Autodesk Inventor part; units mm, degrees
ref_plane "YZ Plane" through (0, 0, 0) normal (1, 0, 0) x (0, 1, 0)
ref_plane "XZ Plane" through (0, 0, 0) normal (0, 1, 0) x (-1, 0, 0)
ref_plane "XY Plane" through (0, 0, 0) normal (0, 0, 1) x (1, 0, 0)
sketch "Sketch1" plane through (0, 0, 0) normal (0, 0, 1) x (1, 0, 0)
  line L0 (49.9396, 9.6174) -> (57.9396, 9.6174)
  line L1 (57.9396, -8.4526) -> (49.9396, -8.4526)
  line L2 (49.9396, -8.4526) -> (49.9396, 9.6174)
  line L3 (57.9396, -8.4526) -> (57.9396, 9.6174)
  line L4 (-49.449, 9.6174) -> (-49.449, -8.4526)
  line L5 (-49.449, -8.4526) -> (-57.449, -8.4526)
  line L6 (-57.449, 9.6174) -> (-57.449, -8.4526)
  line L7 (-45.5464, 0.7392) -> (-34.5464, 0.7392)
  line L8 (-33.5464, 1.7392) -> (-33.5464, 6.2392)
  line L9 (-34.5464, 7.2392) -> (-45.5464, 7.2392)
  line L10 (-46.5464, 6.2392) -> (-46.5464, 1.7392)
  line L11 (-30.5291, -2.0275) -> (3.4709, -2.0275)
  line L12 (4.4709, -1.0275) -> (4.4709, 3.9725)
  line L13 (-31.5291, 3.9725) -> (-31.5291, -1.0275)
  circle A0 centre (-88.9996, -15.383) radius 1.5
  circle A1 centre (-64.9996, -15.383) radius 1.5
  circle A2 centre (-64.9996, 8.617) radius 1.5
  circle A3 centre (-88.9996, 8.617) radius 1.5
  arc A4 (-82.1595, 3.0543) -> (-82.1595, -9.8202) centre (-76.9996, -3.383) ccw
  arc A5 (-79.9944, -11.0702) -> (-68.8448, -4.633) centre (-76.9996, -3.383) ccw
  arc A6 (-68.8448, -2.133) -> (-79.9944, 4.3043) centre (-76.9996, -3.383) ccw
  arc A7 (-82.0034, -16.8856) -> (-62.804, -5.8009) centre (-76.9996, -3.383) ccw
  arc A8 (-63.7898, -2.133) -> (-62.804, -0.9651) centre (-63.7898, -1.133) ccw
  arc A9 (-62.804, -0.9651) -> (-82.0034, 10.1197) centre (-76.9996, -3.383) ccw
  arc A10 (-82.0034, 10.1197) -> (-82.5219, 8.682) centre (-81.6559, 9.182) ccw
  line L14 (-82.5219, 8.682) -> (-79.9944, 4.3043)
  line L15 (-82.1595, 3.0543) -> (-84.687, 7.432)
  arc A11 (-84.687, 7.432) -> (-86.1913, 7.7018) centre (-85.553, 6.932) ccw
  arc A12 (-86.1913, 7.7018) -> (-86.1913, -14.4677) centre (-76.9996, -3.383) ccw
  arc A13 (-86.1913, -14.4677) -> (-84.687, -14.1979) centre (-85.553, -13.6979) ccw
  line L16 (-84.687, -14.1979) -> (-82.1595, -9.8202)
  arc A14 (-82.5219, -15.4479) -> (-82.0034, -16.8856) centre (-81.6559, -15.9479) ccw
  line L17 (-79.9944, -11.0702) -> (-82.5219, -15.4479)
  line L18 (-63.7898, -4.633) -> (-68.8448, -4.633)
  arc A15 (-62.804, -5.8009) -> (-63.7898, -4.633) centre (-63.7898, -5.633) ccw
  line L19 (-68.8448, -2.133) -> (-63.7898, -2.133)
  circle A16 centre (64.9975, -15.3839) radius 1.5
  circle A17 centre (88.9975, -15.3839) radius 1.5
  circle A18 centre (88.9975, 8.6161) radius 1.5
  circle A19 centre (64.9975, 8.6161) radius 1.5
  line L20 (71.4751, 8.6811) -> (74.0026, 4.3033)
  arc A20 (71.9936, 10.1188) -> (71.4751, 8.6811) centre (72.3411, 9.1811) ccw
  arc A21 (91.193, -0.966) -> (71.9936, 10.1188) centre (76.9975, -3.3839) ccw
  arc A22 (85.1522, -2.1339) -> (74.0026, 4.3033) centre (76.9975, -3.3839) ccw
  line L21 (85.1522, -2.1339) -> (90.2072, -2.1339)
  arc A23 (90.2072, -2.1339) -> (91.193, -0.966) centre (90.2072, -1.1339) ccw
  arc A24 (91.193, -5.8018) -> (90.2072, -4.6339) centre (90.2072, -5.6339) ccw
  arc A25 (71.9936, -16.8866) -> (91.193, -5.8018) centre (76.9975, -3.3839) ccw
  arc A26 (74.0026, -11.0711) -> (85.1522, -4.6339) centre (76.9975, -3.3839) ccw
  line L22 (74.0026, -11.0711) -> (71.4751, -15.4489)
  line L23 (69.31, -14.1989) -> (71.8375, -9.8211)
  arc A27 (67.8057, -14.4686) -> (69.31, -14.1989) centre (68.444, -13.6989) ccw
  arc A28 (67.8057, 7.7009) -> (67.8057, -14.4686) centre (76.9975, -3.3839) ccw
  arc A29 (71.8375, 3.0533) -> (71.8375, -9.8211) centre (76.9975, -3.3839) ccw
  line L24 (71.8375, 3.0533) -> (69.31, 7.4311)
  arc A30 (69.31, 7.4311) -> (67.8057, 7.7009) centre (68.444, 6.9311) ccw
  arc A31 (71.4751, -15.4489) -> (71.9936, -16.8866) centre (72.3411, -15.9489) ccw
  line L25 (90.2072, -4.6339) -> (85.1522, -4.6339)
  line L26 (-49.449, 9.6174) -> (-57.449, 9.6174)
  line L27 (3.4709, 4.9725) -> (-30.5291, 4.9725)
  arc A32 (-34.5464, 0.7392) -> (-33.5464, 1.7392) centre (-34.5464, 1.7392) ccw
  arc A33 (-33.5464, 6.2392) -> (-34.5464, 7.2392) centre (-34.5464, 6.2392) ccw
  arc A34 (-45.5464, 7.2392) -> (-46.5464, 6.2392) centre (-45.5464, 6.2392) ccw
  arc A35 (-46.5464, 1.7392) -> (-45.5464, 0.7392) centre (-45.5464, 1.7392) ccw
  arc A36 (-31.5291, -1.0275) -> (-30.5291, -2.0275) centre (-30.5291, -1.0275) ccw
  arc A37 (-30.5291, 4.9725) -> (-31.5291, 3.9725) centre (-30.5291, 3.9725) ccw
  arc A38 (4.4709, 3.9725) -> (3.4709, 4.9725) centre (3.4709, 3.9725) ccw
  arc A39 (3.4709, -2.0275) -> (4.4709, -1.0275) centre (3.4709, -1.0275) ccw
  line L28 (-57.412, 19.6174) -> (-87.412, 19.6174)
  line L29 (-87.412, 19.6174) -> (-87.412, 24.6174)
  line L30 (-57.412, 24.6174) -> (-87.412, 24.6174)
  line L31 (-57.412, 19.6174) -> (-57.412, 24.6174)
  line L32 (27.588, 19.6174) -> (-27.412, 19.6174)
  line L33 (-27.412, 19.6174) -> (-27.412, 24.6174)
  line L34 (27.588, 24.6174) -> (-27.412, 24.6174)
  line L35 (27.588, 19.6174) -> (27.588, 24.6174)
  line L36 (87.588, 19.6174) -> (57.588, 19.6174)
  line L37 (57.588, 19.6174) -> (57.588, 24.6174)
  line L38 (87.588, 24.6174) -> (57.588, 24.6174)
  line L39 (87.588, 19.6174) -> (87.588, 24.6174)
  line L40 (94.088, -10.3826) -> (94.088, -25.3826)
  line L41 (99.088, -10.3826) -> (94.088, -10.3826)
  line L42 (99.088, 9.6181) -> (99.088, -10.3826)
  line L43 (99.088, 9.6181) -> (94.088, 9.6181)
  line L44 (94.088, 24.6181) -> (94.088, 9.6181)
  line L45 (99.088, 24.6181) -> (94.088, 24.6181)
  line L46 (99.088, 32.6174) -> (99.088, 24.6181)
  line L47 (-98.912, 32.6174) -> (-98.912, 24.6181)
  line L48 (-93.912, 24.6181) -> (-98.912, 24.6181)
  line L49 (-93.912, 24.6181) -> (-93.912, 9.6181)
  line L50 (-93.912, 9.6181) -> (-98.912, 9.6181)
  line L51 (-98.912, 9.6181) -> (-98.912, -10.3826)
  line L52 (-93.912, -10.3826) -> (-98.912, -10.3826)
  line L53 (-93.912, -10.3826) -> (-93.912, -25.3826)
  line L54 (-98.912, 32.6174) -> (99.088, 32.6174)
  line L55 (-93.912, -25.3826) -> (94.088, -25.3826)
  arc A40 (15.5314, -3.6707) -> (16.5314, -2.6707) centre (15.5314, -2.6707) ccw
  arc A41 (16.5314, 5.8293) -> (15.5314, 6.8293) centre (15.5314, 5.8293) ccw
  line L56 (5.7314, -2.6707) -> (5.7314, 5.8293)
  arc A42 (5.7314, -2.6707) -> (6.7314, -3.6707) centre (6.7314, -2.6707) ccw
  arc A43 (6.7314, 6.8293) -> (5.7314, 5.8293) centre (6.7314, 5.8293) ccw
  line L57 (6.7314, 6.8293) -> (15.5314, 6.8293)
  line L58 (6.7314, -3.6707) -> (15.5314, -3.6707)
  line L59 (23.4252, 0.4179) -> (23.4252, -9.0821)
  line L60 (37.4252, 1.4179) -> (24.4252, 1.4179)
  line L61 (24.4252, -10.0821) -> (37.4252, -10.0821)
  line L62 (38.4252, -9.0821) -> (38.4252, 0.4179)
  line L63 (16.5314, -2.6707) -> (16.5314, 5.8293)
  arc A44 (24.4252, 1.4179) -> (23.4252, 0.4179) centre (24.4252, 0.4179) ccw
  arc A45 (23.4252, -9.0821) -> (24.4252, -10.0821) centre (24.4252, -9.0821) ccw
  arc A46 (37.4252, -10.0821) -> (38.4252, -9.0821) centre (37.4252, -9.0821) ccw
  arc A47 (38.4252, 0.4179) -> (37.4252, 1.4179) centre (37.4252, 0.4179) ccw
  point P0 (-50.5662, -19.8134)
  point P1 (94.0004, -33.3808)
  point P2 (-46.5464, 0.7392)
  point P3 (-33.5464, 7.2392)
  point P4 (-33.5464, 0.7392)
  point P5 (-46.5464, 7.2392)
  point P6 (-31.5291, -2.0275)
  point P7 (4.4709, 4.9725)
  point P8 (4.4709, -2.0275)
  point P9 (-31.5291, 4.9725)
  point P10 (3.4709, -1.0275)
  point P11 (23.4252, 1.4179)
  point P12 (5.7314, -3.6707)
  point P13 (16.5314, 6.8293)
  point P14 (16.5314, -3.6707)
  point P15 (23.4252, -10.0821)
  point P16 (38.4252, -10.0821)
  point P17 (38.4252, 1.4179)
  dimension "d20" = 8
  dimension "d47" = 8
  dimension "d53" = 6.5
  dimension "d54" = 13
  dimension "d56" = 36
  dimension "d59" = 1
  dimension "d60" = 7
  dimension "d73" = 10.5
  dimension "d74" = 10.8
  dimension "d75" = 11.5
  dimension "d76" = 15
extrude "Extrusion2" add sketch "Sketch1" along normal blind 5
sketch "Sketch2" plane through (0, 0, 0) normal (0, 0, -1) x (-1, 0, 0)
  line L0 (92.3846, -19.3253) -> (61.6146, -19.3253)
  line L1 (61.6146, -19.3253) -> (61.6146, 12.5593)
  line L2 (61.6146, 12.5593) -> (92.3846, 12.5593)
  line L3 (92.3846, 12.5593) -> (92.3846, -19.3253)
  arc A0 (82.1595, -9.8202) -> (82.1595, 3.0543) centre (76.9996, -3.383) ccw
  line L4 (92.3846, -19.3253) -> (61.6146, 12.5593) construction
  line L5 (61.6146, -19.3253) -> (92.3846, 12.5593) construction
  line L6 (-61.3514, -21.1002) -> (-92.6435, -21.1002)
  line L7 (-92.6435, -21.1002) -> (-92.6435, 14.3324)
  line L8 (-92.6435, 14.3324) -> (-61.3514, 14.3324)
  line L9 (-61.3514, 14.3324) -> (-61.3514, -21.1002)
  arc A1 (-67.8057, -14.4686) -> (-67.8057, 7.7009) centre (-76.9975, -3.3839) ccw
  line L10 (-61.3514, -21.1002) -> (-92.6435, 14.3324) construction
  line L11 (-92.6435, -21.1002) -> (-61.3514, 14.3324) construction
  point P0 (0, 0)
extrude "Extrusion3" add sketch "Sketch2" against normal blind 5
sketch "Sketch3" plane through (0, 0, 0) normal (0, 0, -1) x (-1, 0, 0)
  line L0 (44.362, -11.7916) -> (-44.638, -11.7916)
  line L1 (-48.638, -7.7916) -> (-48.638, 6.2084)
  line L2 (-44.638, 10.2084) -> (44.362, 10.2084)
  line L3 (48.362, 6.2084) -> (48.362, -7.7916)
  line L4 (48.362, -11.7916) -> (-48.638, 10.2084) construction
  line L5 (-48.638, -11.7916) -> (48.362, 10.2084) construction
  arc A0 (44.362, -11.7916) -> (48.362, -7.7916) centre (44.362, -7.7916) ccw
  arc A1 (-48.638, -7.7916) -> (-44.638, -11.7916) centre (-44.638, -7.7916) ccw
  arc A2 (-44.638, 10.2084) -> (-48.638, 6.2084) centre (-44.638, 6.2084) ccw
  arc A3 (48.362, 6.2084) -> (44.362, 10.2084) centre (44.362, 6.2084) ccw
  line L6 (-99.088, -10.3826) -> (-99.088, 9.6181)
  line L7 (-99.088, 32.6174) -> (98.912, 32.6174)
  line L8 (98.912, 9.6181) -> (98.912, -10.3826)
  point P0 (0, 0)
  point P1 (-0.138, -0.7916)
  point P2 (-48.638, -0.7916)
  dimension "d79" = 97
  dimension "d80" = 22
  dimension "d81" = 4
  dimension "d83" = 22.409
  dimension "d84" = 50.55
extrude "Extrusion4" cut sketch "Sketch3" against normal blind 5
properties part number "case top back" material "Lead"
Here's how the part is built. I have some questions about the finished solid (model axes, mm). A direction names the side the tool comes from. Give positions to 0.01 mm unless a question says otherwise; leave off trailing zeros. Loops run counter-clockwise (first coordinate to the right, second up) from the corner with the lowest first, then second, coordinate; pieces in that order, holes last. Notation, with made-up numbers: M 36,21.5 L 82,21.5 A12 cw 82,42.5 Z; hole C 24,49 d6. An arc over 180 degrees is marked long. Use one line per item in the form item = value. Start each with the question number.
Q1. If we section it at C-C (x = -13.5): Write out the boundary of the cut face in (y, z).
Q2. Which directions (+Z, -Z, +X, -X, +Y, -Y) give clear straight access to the entire face, cutting with the end or side of a thin tool? Please do faces 4 (the flat face through (48.638, -1, 2)), 5 (the flat face through (-98.912, 29, 2)), 6 (the flat face through (97, 9.618, 2)).
Q3. If we section it at A-A (y = 2): Write out the boundary of the cut face in (x, z).
Q4. Will these pins go through, and if not, where does the flat tip stop? pin 1 Ø1.5 at (y, z) = (23, 3) entering from +X; pin 2 Ø1.5 at (y, z) = (16.5, 2) entering from -X; pin 3 Ø2 at (x, y) = (-31, -9) entering from +Z; pin 4 Ø2.5 at (x, z) = (-96, 3.5) entering from -Y.
Q5. Thinking about a two-plate mould opening in X: for faces 1 (the flat face through (-49.449, 1, 2)), 2 (the flat face through (-1.3, 10.5, 5)), 3 (the flat face through (94.088, 17, 2)), which applies, +X half, -X half, draft (parallel to the pull), parting line (faces both ways), or undercut?
Q6. If we section it at D-D (x = -52.5): Write out the boundary of the cut face in (y, z), then the cut area to 3 significant figures.
Q7. If we section it at B-B (x = 42.5): Write out the boundary of the cut face in (y, z), then the cut area to 3 significant figures.
Q8. I need wall thicknesses on line 1 along Y through (x, z) = (-8, 4.4); line 2 along X through (y, z) = (-6.5, 2.35); line 3 along X through (y, z) = (21.5, 3). Which ranges of each line are inside material? Lowest first, please.
Taken from the geometry:
q1.outline = M -25.38,0 L -11.79,0 L -11.79,5 L -25.38,5 Z; M 10.21,0 L 19.62,0 L 19.62,5 L 10.21,5 Z; M 24.62,0 L 32.62,0 L 32.62,5 L 24.62,5 Z
q2.face_4 = +Z, -Z
q2.face_5 = +Z, -Z, -X, +Y, -Y
q2.face_6 = +Z, -Z, +X
q3.outline = M -98.91,0 L -57.45,0 L -57.45,5 L -98.91,5 Z; M -49.45,0 L -48.36,0 L -48.36,5 L -49.45,5 Z; M 48.64,0 L 49.94,0 L 49.94,5 L 48.64,5 Z; M 57.94,0 L 99.09,0 L 99.09,5 L 57.94,5 Z
q4.pin_1 = 94.09
q4.pin_2 = -93.91
q4.pin_3 = through
q4.pin_4 = -10.38
q5.face_1 = undercut
q5.face_2 = draft
q5.face_3 = +X half
q6.outline = M -25.38,0 L -8.45,0 L -8.45,5 L -25.38,5 Z; M 9.62,0 L 32.62,0 L 32.62,5 L 9.62,5 Z
q6.area = 200 mm^2
q7.outline = M -25.38,0 L -11.79,0 L -11.79,5 L -25.38,5 Z; M 10.21,0 L 32.62,0 L 32.62,5 L 10.21,5 Z
q7.area = 180 mm^2
q8.line_1 = -25.38 to -11.79, 10.21 to 19.62, 24.62 to 32.62
q8.line_2 = -98.91 to -57.45, -49.45 to -48.36, 48.64 to 49.94, 57.94 to 99.09
q8.line_3 = -93.91 to -87.41, -57.41 to -27.41, 27.59 to 57.59, 87.59 to 94.09
